```python
from build123d import *

# Parameters (mm, degrees)
SKETCH1_R           = 28
BOSS_EXTRUDE1_DEPTH = 4
BOSS_EXTRUDE2_DEPTH = 2.5
CUT_EXTRUDE1_DEPTH  = 2.5
CUT_EXTRUDE2_DEPTH  = 7.5
SKETCH5_R           = 1.7
CUT_EXTRUDE3_DEPTH  = 5
SKETCH7_OUTSIDE_W   = 88.892
SKETCH7_OUTSIDE_H   = 88.892
CUT_EXTRUDE4_DEPTH  = 7.5
CUT_EXTRUDE4_TAPER  = 45


with BuildPart() as part:
    # Sketch1 → Boss-Extrude1 (new body)
    with BuildSketch(Plane.XY):
        Circle(SKETCH1_R)
    extrude(amount=BOSS_EXTRUDE1_DEPTH)

    # Sketch2 → Boss-Extrude2 (add)
    with BuildSketch(Plane(origin=(0, 0, 0), x_dir=(-1, 0, 0), z_dir=(0, 0, -1))):
        with BuildLine():
            Line((-7.348469228, -6), (7.348469228, -6))
            ThreePointArc((7.348469228, -6), (8.737199378, -6.93305329), (8.398250547, -8.571428571))
            ThreePointArc((8.398250547, -8.571428571), (0, -12), (-8.398250547, -8.571428571))
            ThreePointArc((-8.398250547, -8.571428571), (-8.737199378, -6.93305329), (-7.348469228, -6))
        make_face()
        with BuildLine():
            Line((7.348469228, 6), (-7.348469228, 6))
            ThreePointArc((-7.348469228, 6), (-8.737199378, 6.93305329), (-8.398250547, 8.571428571))
            ThreePointArc((-8.398250547, 8.571428571), (0, 12), (8.398250547, 8.571428571))
            ThreePointArc((8.398250547, 8.571428571), (8.737199378, 6.93305329), (7.348469228, 6))
        make_face()
    extrude(amount=BOSS_EXTRUDE2_DEPTH)

    # Sketch3 → Cut-Extrude1 (cut)
    with BuildSketch(Plane.XY.offset(4)):
        with BuildLine():
            Line((-17.5, 4.75), (-17.5, -4.75))
            ThreePointArc((-17.5, -4.75), (-17.060660172, -5.810660172), (-16, -6.25))
            Line((-16, -6.25), (-13.765564437, -6.25))
            ThreePointArc((-13.765564437, -6.25), (-13.483765285, -6.290526583), (-13.224806846, -6.408821525))
            Line((-13.224806846, -6.408821525), (-10.218918256, -8.341178475))
            ThreePointArc((-10.218918256, -8.341178475), (-9.959959817, -8.459473417), (-9.678160664, -8.5))
            Line((-9.678160664, -8.5), (9.734435563, -8.5))
            ThreePointArc((9.734435563, -8.5), (10.018134319, -8.458913456), (10.278520672, -8.339030031))
            Line((10.278520672, -8.339030031), (13.251769281, -6.410969969))
            ThreePointArc((13.251769281, -6.410969969), (13.512155635, -6.291086544), (13.795854391, -6.25))
            Line((13.795854391, -6.25), (16, -6.25))
            ThreePointArc((16, -6.25), (17.060660172, -5.810660172), (17.5, -4.75))
            Line((17.5, -4.75), (17.5, 4.75))
            ThreePointArc((17.5, 4.75), (17.060660172, 5.810660172), (16, 6.25))
            Line((16, 6.25), (13.793701886, 6.25))
            ThreePointArc((13.793701886, 6.25), (13.511902734, 6.290526583), (13.252944295, 6.408821525))
            Line((13.252944295, 6.408821525), (10.247055705, 8.341178475))
            ThreePointArc((10.247055705, 8.341178475), (9.988097266, 8.459473417), (9.706298114, 8.5))
            Line((9.706298114, 8.5), (-9.704145609, 8.5))
            ThreePointArc((-9.704145609, 8.5), (-9.987844365, 8.458913456), (-10.248230719, 8.339030031))
            Line((-10.248230719, 8.339030031), (-13.221479328, 6.410969969))
            ThreePointArc((-13.221479328, 6.410969969), (-13.481865681, 6.291086544), (-13.765564437, 6.25))
            Line((-13.765564437, 6.25), (-16, 6.25))
            ThreePointArc((-16, 6.25), (-17.060660172, 5.810660172), (-17.5, 4.75))
        make_face()
    extrude(amount=-CUT_EXTRUDE1_DEPTH, mode=Mode.SUBTRACT)

    # Sketch4 → Cut-Extrude2 (cut, through all)
    with BuildSketch(Plane(origin=(0, 0, -2.5), x_dir=(-1, 0, 0), z_dir=(0, 0, -1))):
        with BuildLine():
            Line((-6.5, -6), (8.5, -6))
            ThreePointArc((8.5, -6), (9.207106781, -5.707106781), (9.5, -5))
            Line((9.5, -5), (9.5, 5))
            ThreePointArc((9.5, 5), (9.207106781, 5.707106781), (8.5, 6))
            Line((8.5, 6), (-6.5, 6))
            ThreePointArc((-6.5, 6), (-8.621320344, 5.121320344), (-9.5, 3))
            Line((-9.5, 3), (-9.5, -3))
            ThreePointArc((-9.5, -3), (-8.621320344, -5.121320344), (-6.5, -6))
        make_face()
    extrude(amount=-CUT_EXTRUDE2_DEPTH, mode=Mode.SUBTRACT)

    # Sketch5 → Cut-Extrude3 (cut, through all)
    with BuildSketch(Plane.XY.offset(1.5)):
        with Locations((-12.5, 0)):
            Circle(SKETCH5_R)
        with Locations((12.5, 0)):
            Circle(SKETCH5_R)
    extrude(amount=-CUT_EXTRUDE3_DEPTH, mode=Mode.SUBTRACT)

    # Sketch7 outside → Cut-Extrude4 (cut, through all)
    with BuildSketch(Plane.XY.offset(4)):
        Rectangle(SKETCH7_OUTSIDE_W, SKETCH7_OUTSIDE_H)
        Polygon((0, 22), (-19.052558883, 11), (-19.052558883, -11), (0, -22), (19.052558883, -11), (19.052558883, 11), align=None, mode=Mode.SUBTRACT)
    extrude(amount=-CUT_EXTRUDE4_DEPTH, taper=CUT_EXTRUDE4_TAPER, mode=Mode.SUBTRACT)


solid = part.part
```
For this review, take the finished solid that the model builds, in its own axes (mm). A direction names the side the tool comes from. Coordinates: 2 decimals unless noted, no trailing zeros. Loops run counter-clockwise (first coordinate to the right, second up) from the corner with the lowest first, then second, coordinate; pieces in that order, holes last.
1. For line 1 (Z direction, x = -3.5, y = 18.5); line 2 (Y direction, x = -12.5, z = 0.75); line 3 (Y direction, x = 12.5, z = 0.9), list the stretches that pass through material, from the lowest coordinate up.
2. Mouldability with a two-part tool opening along Y and no side actions: class faces 4 (the flat face through (-15, 6.25, 3)), 5 (the flat face through (0, 8, -2.5)), 6 (the cylindrical face through (-8.728, -6.91, -1.232)) as +Y half, -Y half, draft (parallel to the pull), parting line (faces both ways), or undercut.
3. Insertion check: P1, Ø4.5, axis at x = 12.5, y = 0, coming from the -Z side; P2, Ø6, axis at x = 10.5, y = 3.5, coming from the +Z side; P3, Ø2, axis at x = -12.5, y = 0, coming from the -Z side; P4, Ø2, axis at x = 3, z = 2, coming from the -Y side. Each pin has a flat end and moves straight along its axis. Give the tip position at first contact, or say it passes through.
4. Add section A-A, the plane z = -1.5. Give the boundary of the cut face in (x, y), then the cut area to 3 significant figures.
5. Add section B-B, the plane y = 0. Count the separate pieces of the cut face and the enclosed holes in it, then the cut area to 3 significant figures.
6. For faces 1 (the flat face through (-10.6, 0.4, 0)), 2 (the cylindrical face through (8.728, 6.91, -1.232)), 3 (the cylindrical face through (17.05, -5.82, 2.77)), list the 3-axis set-ups (+Z, -Z, +X, -X, +Y, -Y) from which the entire face can be reached by the end or side of a thin tool; tool diameter is ignored.
Result:
1. line 1: z = 0 to 4
1. line 2: y = -18.54 to -1.7, 1.7 to 18.54
1. line 3: y = -18.36 to -1.7, 1.7 to 18.36
2. face 4: undercut
2. face 5: draft
2. face 6: undercut
3. P1: stops at z = 0
3. P2: stops at z = 1.5
3. P3: passes through
3. P4: stops at y = -23.87
4. outline: (-8.4, -8.57) arc R12 ccw to (8.4, -8.57) arc R1.5 ccw to (7.35, -6) - (-7.35, -6) arc R1.5 ccw to start; (-8.4, 8.57) arc R1.5 ccw to (-7.35, 6) - (7.35, 6) arc R1.5 ccw to (8.4, 8.57) arc R12 ccw to start
4. area: 168 mm2
5. separate pieces: 4
5. enclosed holes: 0
5. area: 42.2 mm2
6. face 1: -Z
6. face 2: -Z, +X
6. face 3: +Z
